Input: part model. Units: mm. Frame: model coordinates. A direction names the side the tool comes from. Coordinates: 2 decimals unless noted, no trailing zeros. Write each loop counter-clockwise with the first axis right and the second up, starting at its lowest first coordinate (ties: lowest second). Pieces come first, ordered by that corner, then holes. Notation, with made-up numbers: (33.25, 16) -> (70.25, 16) arc R23 ccw to (70.25, 47) -> close; hole circle Ø9 at (3.5, 61.25). An arc over 180 degrees is marked (long way). One line per question, with ' | ' between items. Start each with the question number.
```python
from build123d import *

# Parameters (mm, degrees)
SKETCH1_R           = 2
SKETCH1_R_2         = 0.75
SKETCH1_W           = 9
SKETCH1_H           = 2
SKETCH1_W_2         = 5
SKETCH1_W_3         = 8
SKETCH1_H_2         = 6
SKETCH1_H_3         = 4
SKETCH1_W_4         = 6
BOSS_EXTRUDE1_DEPTH = 4


with BuildPart() as part:
    # Sketch1 → Boss-Extrude1 (new body)
    with BuildSketch(Plane.XY):
        with BuildLine():
            Line((-0.718612481, -17.999985362), (-0.718612481, -23.999985362))
            Line((-0.718612481, -23.999985362), (35.281387519, -23.999985362))
            Line((35.281387519, -23.999985362), (35.281387519, -17.999985362))
            ThreePointArc((35.281387519, -17.999985362), (42.406223237, -14.93064645), (47.407370228, -8.999992681))
            ThreePointArc((47.407370228, -8.999992681), (58.276211887, 27.829327454), (55.330365794, 66.115781082))
            Line((55.330365794, 66.115781082), (39.484374663, 69.483950474))
            Line((39.484374663, 69.483950474), (38.221859922, 75.558279649))
            Line((38.221859922, 75.558279649), (22.02432726, 75.841009004))
            Line((22.02432726, 75.841009004), (19.881449124, 82.510000006))
            Line((19.881449124, 82.510000006), (3.681449124, 82.510000006))
            Line((3.681449124, 82.510000006), (-2.261308264, 82.298430785))
            Line((-2.261308264, 82.298430785), (-18.458840926, 82.015701198))
            ThreePointArc((-18.458840926, 82.015701198), (-20.226607879, 81.283468151), (-20.958840926, 79.515701198))
            ThreePointArc((-20.958840926, 79.515701198), (-22.767055021, 46.485509252), (-23.410346484, 13.412115197))
            ThreePointArc((-23.410346484, 13.412115197), (-19.613036862, 1.256548647), (-12.064479482, -8.999992681))
            ThreePointArc((-12.064479482, -8.999992681), (-6.700212214, -13.889110006), (-0.718612481, -17.999985362))
        make_face()
        with Locations((50.407370195, 11.821617405)):
            Circle(SKETCH1_R, mode=Mode.SUBTRACT)
        with Locations((-1.739971548, -9.124358763)):
            Circle(SKETCH1_R, mode=Mode.SUBTRACT)
        with Locations((6.531449125, 80.01)):
            Circle(SKETCH1_R_2, mode=Mode.SUBTRACT)
        with Locations((-19.42147321, 43.456405989)):
            Circle(SKETCH1_R, mode=Mode.SUBTRACT)
        with Locations(Location((17.031449125, 80.01, 0), (0, 0, 180))):
            Circle(SKETCH1_R_2, mode=Mode.SUBTRACT)
        with Locations(Location((17.031449125, 74.01, 0), (0, 0, 180))):
            Circle(SKETCH1_R_2, mode=Mode.SUBTRACT)
        with Locations((6.531449125, 74.01)):
            Circle(SKETCH1_R_2, mode=Mode.SUBTRACT)
        with Locations((-15.833929885, 79.558146704)):
            Circle(SKETCH1_R_2, mode=Mode.SUBTRACT)
        with Locations(Location((-5.335529086, 79.741396971, 0), (0, 0, 180))):
            Circle(SKETCH1_R_2, mode=Mode.SUBTRACT)
        with Locations((-15.729215446, 73.559060533)):
            Circle(SKETCH1_R_2, mode=Mode.SUBTRACT)
        with Locations(Location((-5.230814647, 73.7423108, 0), (0, 0, 180))):
            Circle(SKETCH1_R_2, mode=Mode.SUBTRACT)
        with Locations(Location((35.223948537, 67.109313963, 0), (0, 0, 180))):
            Circle(SKETCH1_R_2, mode=Mode.SUBTRACT)
        with Locations((24.725547738, 67.29256423)):
            Circle(SKETCH1_R_2, mode=Mode.SUBTRACT)
        with Locations(Location((35.328662975, 73.108400134, 0), (0, 0, 180))):
            Circle(SKETCH1_R_2, mode=Mode.SUBTRACT)
        with Locations((24.830262176, 73.291650401)):
            Circle(SKETCH1_R_2, mode=Mode.SUBTRACT)
        with Locations((40.448000847, 60.683603476)):
            Circle(SKETCH1_R_2, mode=Mode.SUBTRACT)
        with Locations(Location((52.028592853, 64.167837794, 0), (0, 0, 180))):
            Circle(SKETCH1_R_2, mode=Mode.SUBTRACT)
        with Locations((41.797707173, 66.529823865)):
            Circle(SKETCH1_R_2, mode=Mode.SUBTRACT)
        with Locations(Location((50.678886527, 58.321617405, 0), (0, 0, 180))):
            Circle(SKETCH1_R_2, mode=Mode.SUBTRACT)
        with Locations((11.781449159, 77.509999643)):
            Rectangle(SKETCH1_W, SKETCH1_H, mode=Mode.SUBTRACT)
        Polygon((2.597827224, 24.068199743), (3.110016694, 28.94135703), (-10.944069886, 30.418501052), (-10.525956033, 34.396588634), (-18.482131196, 35.23281634), (-18.900245049, 31.254728759), (-21.883810735, 31.568314148), (-22.396000205, 26.695156861), (-19.412434519, 26.381571471), (-19.830548372, 22.40348389), (-11.874373209, 21.567256184), (-11.456259356, 25.545343765), align=None, mode=Mode.SUBTRACT)
        with BuildLine():
            Line((22.61884629, 63.151218734), (22.61884629, 60.151218734))
            Line((22.61884629, 60.151218734), (20.61884629, 60.151218734))
            ThreePointArc((20.61884629, 60.151218734), (6.781449125, 61.651218734), (20.61884629, 63.151218734))
            Line((20.61884629, 63.151218734), (22.61884629, 63.151218734))
        make_face(mode=Mode.SUBTRACT)
        with Locations((47.407370195, 56.321617405)):
            Rectangle(SKETCH1_W_2, SKETCH1_H, mode=Mode.SUBTRACT)
        with BuildLine():
            Line((-5.581534458, 63.151218734), (-3.581534458, 63.151218734))
            Line((-3.581534458, 63.151218734), (-3.581534458, 60.151218734))
            Line((-3.581534458, 60.151218734), (-5.581534458, 60.151218734))
            ThreePointArc((-5.581534458, 60.151218734), (-19.418931624, 61.651218734), (-5.581534458, 63.151218734))
        make_face(mode=Mode.SUBTRACT)
        Polygon((-15.057865504, 78.071464466), (-6.059236247, 78.228536124), (-6.024331434, 76.228840733), (-15.022960691, 76.071769076), align=None, mode=Mode.SUBTRACT)
        with Locations((-1.794306623, 49.875576367)):
            Rectangle(SKETCH1_W_3, SKETCH1_H_2, mode=Mode.SUBTRACT)
        with Locations((30.123093592, 56.321617405)):
            Rectangle(SKETCH1_W_2, SKETCH1_H, mode=Mode.SUBTRACT)
        with Locations((11.781449125, 71.151218734)):
            Rectangle(SKETCH1_W_2, SKETCH1_H, mode=Mode.SUBTRACT)
        Polygon((25.553969338, 71.778789554), (25.519064525, 69.779094163), (34.517693781, 69.622022505), (34.552598594, 71.621717896), align=None, mode=Mode.SUBTRACT)
        with BuildLine():
            Line((20.285696426, 48.321617405), (18.285696426, 48.321617405))
            Line((18.285696426, 48.321617405), (18.285696426, 45.321617405))
            Line((18.285696426, 45.321617405), (20.285696426, 45.321617405))
            ThreePointArc((20.285696426, 45.321617405), (34.123093592, 46.821617405), (20.285696426, 48.321617405))
        make_face(mode=Mode.SUBTRACT)
        Polygon((50.960388723, 62.874995987), (42.19105814, 64.899555477), (41.741156031, 62.950815347), (50.510486614, 60.926255858), align=None, mode=Mode.SUBTRACT)
        with BuildLine():
            Line((41.569973029, 45.321617405), (43.569973029, 45.321617405))
            ThreePointArc((43.569973029, 45.321617405), (57.407370195, 46.821617405), (43.569973029, 48.321617405))
            Line((43.569973029, 48.321617405), (41.569973029, 48.321617405))
            Line((41.569973029, 48.321617405), (41.569973029, 45.321617405))
        make_face(mode=Mode.SUBTRACT)
        with Locations((-10.418931624, 71.151218734)):
            Rectangle(SKETCH1_W_2, SKETCH1_H, mode=Mode.SUBTRACT)
        Polygon((8.260028452, -2.5), (12.260028452, -2.5), (12.260028452, 0), (24.260028452, 0), (24.260028452, -2.5), (28.260028452, -2.5), (28.260028452, -12.5), (24.260028452, -12.5), (24.260028452, -15), (12.260028452, -15), (12.260028452, -12.5), (8.260028452, -12.5), align=None, mode=Mode.SUBTRACT)
        with Locations((-12.294306623, 51.875576367)):
            Rectangle(SKETCH1_W_2, SKETCH1_H, mode=Mode.SUBTRACT)
        with Locations((-1.794306623, -0.124358763)):
            Rectangle(SKETCH1_W_3, SKETCH1_H_3, mode=Mode.SUBTRACT)
        with Locations((-12.294306623, -1.124358763)):
            Rectangle(SKETCH1_W_2, SKETCH1_H, mode=Mode.SUBTRACT)
        Polygon((14.723408467, 21.026286371), (13.223408467, 23.624362582), (10.223408467, 23.624362582), (8.723408467, 21.026286371), (10.223408467, 18.428210159), (13.223408467, 18.428210159), align=None, mode=Mode.SUBTRACT)
        with Locations((10.223408467, 8.717005814)):
            Rectangle(SKETCH1_W_4, SKETCH1_H_3, mode=Mode.SUBTRACT)
        with Locations((10.223408467, 33.335566927)):
            Rectangle(SKETCH1_W_4, SKETCH1_H_3, mode=Mode.SUBTRACT)
        with Locations((-12.294306623, 8.717005814)):
            Rectangle(SKETCH1_W_2, SKETCH1_H_3, mode=Mode.SUBTRACT)
        with Locations((-12.294306623, 40.719533555)):
            Rectangle(SKETCH1_W_2, SKETCH1_H_3, mode=Mode.SUBTRACT)
    extrude(amount=BOSS_EXTRUDE1_DEPTH)


solid = part.part
```
1) Pull-direction query (X, two-part tool) for faces 3 (the face through (-22.75, 46.95, 1.97)), 4 (the face through (-2, -2.124, 2)); classes: released by +X, released by -X, zero draft, split by the parting line, or undercut.
2) Access query for faces 1 (the face through (-6.78, -13.826, 1.972)), 2 (the face through (22.619, 62, 2)). Directions: +Z, -Z, +X, -X, +Y, -Y. A direction counts if a zero-diameter tool reaches every point of the face in a straight line with its end or side. Return the directions, or none.
3) Ray query, line 1 (Y direction, x = -15.5, z = 2.4); line 2 (Y direction, x = 8.5, z = 1.45); line 3 (X direction, y = -1, z = 0.4). Return the intervals inside material, ascending.
4) Section B-B, the plane y = 15. Return loops of the section in (x, z).
5) First-contact query: P1, Ø1.2, axis at x = -5.34, y = 79.74, coming from the +Z side; P2, Ø1.2, axis at y = 32.5, z = 1.5, coming from the +X side; P3, Ø2, axis at y = 56, z = 2, coming from the -X side; P4, Ø2.5, axis at x = 35.22, y = 67.11, coming from the -Z side. Flat tips, straight axial feed; report the tip coordinate or a pass-through.
6) Section A-A, the plane z = 2.55. Give the number of separate pieces and of enclosed holes in the cut face, then the cut area to 3 significant figures.
Answer block:
1) face 3: released by -X | face 4: undercut
2) face 1: +Z, -Z, -X, -Y | face 2: +Z, -Z
3) line 1: y = -5.19 to 21.95, 34.92 to 55.37, 67.94 to 72.84, 74.27 to 78.89, 80.23 to 82.07 | line 2: y = -24 to -12.5, -2.5 to 6.72, 10.72 to 31.34, 35.34 to 57.06, 66.25 to 76.51, 78.51 to 82.51 | line 3: x = -18.37 to -14.79, -9.79 to -5.79, 2.21 to 12.26, 24.26 to 51.05
4) outline: (-23.41, 0) -> (56.12, 0) -> (56.12, 4) -> (-23.41, 4) -> close
5) P1: passes through | P2: stops at x = 58.7 | P3: stops at x = -22.41 | P4: stops at z = 0
6) separate pieces: 1 | enclosed holes: 42 | area: 5,930 mm2
